Build history of the part. All positions in model axes, mm. Face numbers are marked on the shaded views. Give positions to 0.01 mm unless a question says otherwise; leave off trailing zeros. Write each loop counter-clockwise with the first axis right and the second up, starting at its lowest first coordinate (ties: lowest second). Pieces come first, ordered by that corner, then holes.
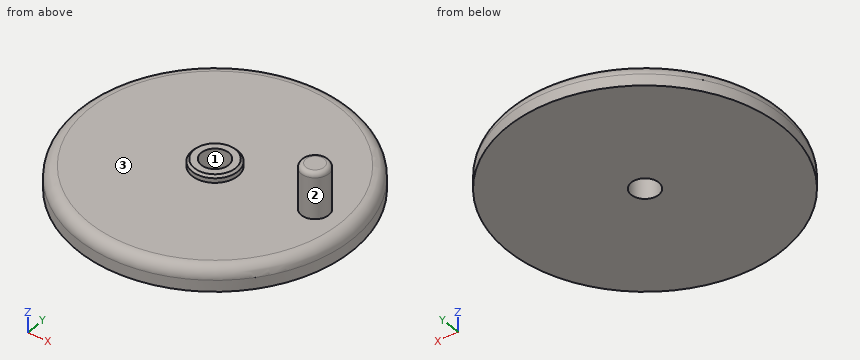
from build123d import *

# Parameters (mm, degrees)
SKETCH1_R           = 60
BOSS_EXTRUDE1_DEPTH = 10
FILLET1_R           = 5
SKETCH2_R           = 10
BOSS_EXTRUDE3_DEPTH = 13
SKETCH2_3_R         = 6
CUT_EXTRUDE1_DEPTH  = 86.842879728
CHAMFER1_SIZE       = 1
SKETCH3_R           = 6
BOSS_EXTRUDE4_DEPTH = 30
FILLET2_R           = 2


with BuildPart() as part:
    # Sketch1 → Boss-Extrude1 (new body)
    with BuildSketch(Plane.XY):
        Circle(SKETCH1_R)
    extrude(amount=BOSS_EXTRUDE1_DEPTH)

    # Fillet1
    fillet1_edges = [part.edges().sort_by_distance(p)[0] for p in [
        (-60, 0, 10),
    ]]
    fillet(fillet1_edges, radius=FILLET1_R)

    # Sketch2 → Boss-Extrude3 (add)
    with BuildSketch(Plane.XY):
        with Locations(Location((0, 0, 0), (0, 0, 180))):
            Circle(SKETCH2_R)
    extrude(amount=BOSS_EXTRUDE3_DEPTH)

    # Sketch2_3 → Cut-Extrude1 (cut, through all)
    with BuildSketch(Plane.XY):
        with Locations(Location((0, 0, 0), (0, 0, 180))):
            Circle(SKETCH2_3_R)
    extrude(amount=CUT_EXTRUDE1_DEPTH, mode=Mode.SUBTRACT)

    # Chamfer1
    chamfer1_edges = [part.edges().sort_by_distance(p)[0] for p in [
        (10, 0, 13),
    ]]
    chamfer(chamfer1_edges, length=CHAMFER1_SIZE)

    # Sketch3 → Boss-Extrude4 (add)
    with BuildSketch(Plane.XY):
        with Locations((43, 0)):
            Circle(SKETCH3_R)
    extrude(amount=BOSS_EXTRUDE4_DEPTH)

    # Fillet2
    fillet2_edges = [part.edges().sort_by_distance(p)[0] for p in [
        (37, 0, 30),
    ]]
    fillet(fillet2_edges, radius=FILLET2_R)


solid = part.part
(1) Saw through at B-B, the plane x = 0. List the corners of the cut face in (y, z).
(2) Probe line 1 (X direction, y = -0.5, z = 5.25); line 2 (Z direction, x = 14, y = -4.5); line 3 (Y direction, x = 0, z = 5.75). List the from-to ranges inside material, lowest first.
(3) Mould opens along Y. For the marked faces 1, 2 and 3 say: +Y half, -Y half, draft (parallel to the pull), parting line (faces both ways), or undercut.
(4) Saw through at A-A, the plane y = 0. List the corners of the cut face in (x, z).
(5) Saw through at C-C, the plane z = 20.75. List the corners of the cut face in (x, y), plus the area to 3 significant figures.
(6) Drop flat-ended pins along their axis: pin 1 (3 mm diameter, centred on x = -3.5, z = 9.5, fed in from -Y); pin 2 (7 mm diameter, centred on x = 0, y = 0, fed in from -Z); pin 3 (20 mm diameter, centred on x = -0.5, y = 1.5, fed in from +Z); pin 4 (6 mm diameter, centred on x = -1.5, z = 14, fed in from -Y). Give the stop position or say it passes through.
Computed values:
1. outline: (-60, 0) - (-6, 0) - (-6, 13) - (-9, 13) - (-10, 12) - (-10, 10) - (-55, 10) arc R5 ccw to (-60, 5) - close; (6, 0) - (60, 0) - (60, 5) arc R5 ccw to (55, 10) - (10, 10) - (10, 12) - (9, 13) - (6, 13) - close
2. line 1: x = -59.99 to -5.98, 5.98 to 59.99
2. line 2: z = 0 to 10
2. line 3: y = -59.94 to -6, 6 to 59.94
3. face 1: undercut
3. face 2: parting line
3. face 3: draft
4. outline: (-60, 0) - (-6, 0) - (-6, 13) - (-9, 13) - (-10, 12) - (-10, 10) - (-55, 10) arc R5 ccw to (-60, 5) - close; (6, 0) - (60, 0) - (60, 5) arc R5 ccw to (55, 10) - (49, 10) - (49, 28) arc R2 ccw to (47, 30) - (39, 30) arc R2 ccw to (37, 28) - (37, 10) - (10, 10) - (10, 12) - (9, 13) - (6, 13) - close
5. outline: circle Ø12 at (43, 0)
5. area: 113 mm2
6. pin 1: stops at y = -58.9
6. pin 2: passes through
6. pin 3: stops at z = 13
6. pin 4: stops at y = -10
